from build123d import *

# Parameters (mm, degrees)
CROQUIS1_W              = 5
CROQUIS1_H              = 2.5
SALIENTE_EXTRUIR1_DEPTH = 5
CROQUIS2_W              = 5
CROQUIS2_H              = 2.5
CROQUIS3_R              = 5.920836197
CROQUIS3_R_2            = 3.60179698
CORTAR_EXTRUIR1_DEPTH   = 5


with BuildPart() as part:
    # Croquis1 → Saliente-Extruir1 (new body)
    with BuildSketch(Plane(origin=(0, 0, 0), x_dir=(1, 0, 0), z_dir=(0, 1, 0))):
        with Locations((2.5, -1.25)):
            Rectangle(CROQUIS1_W, CROQUIS1_H)
    extrude(amount=SALIENTE_EXTRUIR1_DEPTH)

    # Barrer1: sweep along a curve in space
    with BuildLine() as barrer1_path:
        Line((2.5, 5, 1.25), (2.5, 35, 1.25))
        Line((2.5, 35, 1.25), (2.5, 40.786690732, 3.042424523))
        ThreePointArc((2.5, 40.786690732, 3.042424523), (2.5, 42.249249584, 3.377603579), (2.5, 43.745495261, 3.490174748))
        Line((2.5, 43.745495261, 3.490174748), (2.5, 44.85405472, 3.490174748))
        ThreePointArc((2.5, 44.85405472, 3.490174748), (2.5, 46.035691189, 3.420116101), (2.5, 47.200770887, 3.2109218))
        Line((2.5, 47.200770887, 3.2109218), (2.5, 51.840205401, 2.090901298))
        ThreePointArc((2.5, 51.840205401, 2.090901298), (2.5, 53.493312159, 1.030472895), (2.5, 54.136190551, -0.825322817))
        Line((2.5, 54.136190551, -0.825322817), (2.5, 54.136190551, -1.378271143))
        ThreePointArc((2.5, 54.136190551, -1.378271143), (2.5, 53.43445816, -3.306473933), (2.5, 51.657546553, -4.33262182))
        Line((2.5, 51.657546553, -4.33262182), (2.5, 46.898351702, -5.172479734))
        ThreePointArc((2.5, 46.898351702, -5.172479734), (2.5, 46.032749508, -5.28653041), (2.5, 45.160498363, -5.324644146))
        Line((2.5, 45.160498363, -5.324644146), (2.5, 44.439340414, -5.324644146))
        ThreePointArc((2.5, 44.439340414, -5.324644146), (2.5, 43.257703945, -5.254585498), (2.5, 42.092624247, -5.045391197))
        Line((2.5, 42.092624247, -5.045391197), (2.5, 35.083797871, -3.353368343))
        Line((2.5, 35.083797871, -3.353368343), (2.5, 0.100918739, -3.353368343))
    # Croquis2 → Barrer1 (sweep)
    with BuildSketch(Plane(origin=(0, 5, 0), x_dir=(1, 0, 0), z_dir=(0, 1, 0))):
        with Locations((2.5, -1.25)):
            Rectangle(CROQUIS2_W, CROQUIS2_H)
    sweep(path=barrer1_path.line, transition=Transition.RIGHT)

    # Croquis3 → Cortar-Extruir1 (cut)
    with BuildSketch(Plane.XZ):
        with Locations((2.5, -1.10179698)):
            Circle(CROQUIS3_R)
        with Locations((2.5, -1.10179698)):
            Circle(CROQUIS3_R_2, mode=Mode.SUBTRACT)
    extrude(amount=-CORTAR_EXTRUIR1_DEPTH, mode=Mode.SUBTRACT)


solid = part.part
For this review, take the finished solid that the model builds, in its own axes (mm). A direction names the side the tool comes from. Give positions to 0.01 mm unless a question says otherwise; leave off trailing zeros. Order: outer loops, then holes, each group sorted by start corner. A loop starts at its lowest first (then second) coordinate and runs counter-clockwise, first axis right, second up. Notation, with made-up numbers: M -36,77.25 L -2,77.25 A25 cw -2,94.25 Z; hole C -26,22 d5. An arc over 180 degrees is marked long. Answer in a Markdown table with one row per item. Add a question column.
(1) Consider section B-B on y = 24.5. State the section outline as (x, z) points, and give its area (3 significant figures).
(2) Consider section A-A on y = 46. State the section outline as (x, z) points, and give its area (3 significant figures).
(3) Mouldability with a two-part tool opening along Y and no side actions: class faces 1 (the face through (3, 44, 2.24)), 2 (the face through (3, 17, -2.103)), 3 (the face through (2.54, 46.16, -6.53)), 4 (the face through (2.54, 43.13, -6.5)) as +Y half, -Y half, draft (parallel to the pull), parting line (faces both ways), or undercut.
(4) For faces 5 (the face through (2.5, 2.5, 2.5)), 6 (the face through (2.465, 43.42, -4.015)), 7 (the face through (0.4, 5, -4.3)), 8 (the face through (3, 18, 0)), 9 (the face through (4.221, 2.516, -4.266)), list the 3-axis set-ups (+Z, -Z, +X, -X, +Y, -Y) from which the entire face can be reached by the end or side of a thin tool; tool diameter is ignored.
(5) Wall thickness on probe 1 along Z at (x, y) = (4.45, 12.5); probe 2 along Z at (x, y) = (0.4, 42.5); probe 3 along Y at (x, z) = (1.3, -1.75): over which ranges is each line inside the solid? List them lowest first. Write a range as [from, to].
(6) For pin 1 (0.6 mm diameter, centred on x = 3.5, z = -1, fed in from -Y); pin 2 (0.5 mm diameter, centred on x = 0.5, z = -4, fed in from -Y); pin 3 (1 mm diameter, centred on x = 1.5, y = 16.5, fed in from +Z), all flat-tipped, find the tip position at first contact; note any pin that passes through.
Evaluation:
| question | item | result |
|---|---|---|
| 1 | outline | M 0,-4.6 L 5,-4.6 L 5,-2.1 L 0,-2.1 Z; M 0,0 L 5,0 L 5,2.5 L 0,2.5 Z |
| 1 | area | 25.0 mm^2 |
| 2 | outline | M 0,-6.54 L 5,-6.54 L 5,-4.03 L 0,-4.03 Z; M 0,2.16 L 5,2.16 L 5,4.68 L 0,4.68 Z |
| 2 | area | 25.1 mm^2 |
| 3 | face 1 | undercut |
| 3 | face 2 | draft |
| 3 | face 3 | +Y half |
| 3 | face 4 | -Y half |
| 4 | face 5 | +Z, -Y |
| 4 | face 6 | +X, -X |
| 4 | face 7 | -Z, -X, -Y |
| 4 | face 8 | +X, -X, -Y |
| 4 | face 9 | -Z, +X, -Y |
| 5 | probe 1 | z = [-4.6, -2.1], [0, 2.5] |
| 5 | probe 2 | z = [-6.41, -3.86], [2.15, 4.67] |
| 5 | probe 3 | y = [52.85, 55.37] |
| 6 | pin 1 | stops at y = 52.88 |
| 6 | pin 2 | stops at y = 0.1 |
| 6 | pin 3 | stops at z = 2.5 |
